Can you work these out from the model? Positions are in its coordinate system, mm. A direction names the side the tool comes from. Coordinates: 2 decimals unless noted, no trailing zeros. Loops run counter-clockwise (first coordinate to the right, second up) from the corner with the lowest first, then second, coordinate; pieces in that order, holes last.
```python
from build123d import *

# Parameters (mm, degrees)
SKETCH1_R               = 8
BOSS_EXTRUDE1_DEPTH     = 1.5
SKETCH2_R               = 6.11
BOSS_EXTRUDE2_DEPTH     = 7
SKETCH4_R               = 8
BOSS_EXTRUDE4_DEPTH     = 7.5
SKETCH6_R               = 4
CUT_EXTRUDE1_DEPTH      = 16
CUT_EXTRUDE2_REACH      = 21.596
CUT_EXTRUDE2_END_RADIUS = 8
SKETCH7_R               = 2.5
CUT_EXTRUDE3_REACH      = 21.596
CUT_EXTRUDE3_END_RADIUS = 8
SKETCH8_R               = 2.5


with BuildPart() as part:
    # Sketch1 → Boss-Extrude1 (new body)
    with BuildSketch(Plane.XY):
        Circle(SKETCH1_R)
    extrude(amount=BOSS_EXTRUDE1_DEPTH)

    # Sketch2 → Boss-Extrude2 (add)
    with BuildSketch(Plane.XY.offset(1.5)):
        Circle(SKETCH2_R)
    extrude(amount=BOSS_EXTRUDE2_DEPTH)

    # Sketch4 → Boss-Extrude4 (add)
    with BuildSketch(Plane.XY.offset(8.5)):
        Circle(SKETCH4_R)
    extrude(amount=BOSS_EXTRUDE4_DEPTH)

    # Sketch6 → Cut-Extrude1 (cut)
    with BuildSketch(Plane.XY.offset(16)):
        Circle(SKETCH6_R)
    extrude(amount=-CUT_EXTRUDE1_DEPTH, mode=Mode.SUBTRACT)

    # Cut-Extrude2: up to this cylinder (the profile starts inside it)
    cut_extrude2_end = Plane(origin=(0, 0, 12.25), z_dir=(0, 0, -1)) * Cylinder(CUT_EXTRUDE2_END_RADIUS, 60.192, mode=Mode.PRIVATE)
    # Sketch7 → Cut-Extrude2 (cut, up to the surface)
    with BuildSketch(Plane.ZY, mode=Mode.PRIVATE) as cut_extrude2_sk1:
        with Locations((12.25, 0)):
            Circle(SKETCH7_R)
    cut_extrude2_tool1 = extrude(cut_extrude2_sk1.sketch, amount=-CUT_EXTRUDE2_REACH, mode=Mode.PRIVATE) & cut_extrude2_end
    add(cut_extrude2_tool1.solids().sort_by_distance((0, 0, 12.25))[0], mode=Mode.SUBTRACT)

    # Cut-Extrude3: up to this cylinder (the profile starts inside it)
    cut_extrude3_end = Plane(origin=(0, 0, 12.25), z_dir=(0, 0, -1)) * Cylinder(CUT_EXTRUDE3_END_RADIUS, 60.192, mode=Mode.PRIVATE)
    # Sketch8 → Cut-Extrude3 (cut, up to the surface)
    with BuildSketch(Plane(origin=(0, 0, 0), x_dir=(0, 0, 1), z_dir=(0, -1, 0)), mode=Mode.PRIVATE) as cut_extrude3_sk1:
        with Locations(Location((12.25, 0, 0), (0, 0, 180))):
            Circle(SKETCH8_R)
    cut_extrude3_tool1 = extrude(cut_extrude3_sk1.sketch, amount=-CUT_EXTRUDE3_REACH, mode=Mode.PRIVATE) & cut_extrude3_end
    add(cut_extrude3_tool1.solids().sort_by_distance((0, 0, 12.25))[0], mode=Mode.SUBTRACT)


solid = part.part
```
(1) If we mould it in two halves opening along Y, with no side actions, what happens to faces 1 (the cylindrical face through (-3.2, -2.4, 8.1)), 2 (the flat face through (-4, -2, 16)), 3 (the cylindrical face through (-1.73, -7.81, 0.74))? For each: released by +Y, released by -Y, zero draft, split by the parting line, or undercut.
Check values:
face 1: undercut
face 2: zero draft
face 3: split by the parting line
(2) I'm going to push flat-ended pins straight in: pin 1 (1 mm diameter, centred on x = 4, z = 10, fed in from -Y); pin 2 (3 mm diameter, centred on y = -5, z = 11.5, fed in from -X); pin 3 (1 mm diameter, centred on y = 4.5, z = 8.5, fed in from -X). Where does each tip first touch, or does it pass through?
Check values:
pin 1: stops at y = -7.19
pin 2: stops at x = -7.19
pin 3: stops at x = -6.93
(3) I want a section at A-A on x = 0. Write out the boundary of the cut face in (y, z).
Check values:
outline: (-8, 0) - (-4, 0) - (-4, 16) - (-8, 16) - (-8, 8.5) - (-6.11, 8.5) - (-6.11, 1.5) - (-8, 1.5) - close; (4, 0) - (8, 0) - (8, 1.5) - (6.11, 1.5) - (6.11, 8.5) - (8, 8.5) - (8, 9.75) - (4, 9.75) - close; (4, 14.75) - (8, 14.75) - (8, 16) - (4, 16) - close
(4) Which directions (+Z, -Z, +X, -X, +Y, -Y) give clear straight access to the entire face, cutting with the end or side of a thin tool? Please do faces 4 (the cylindrical face through (5.53, -2.44, 11.71)), 5 (the cylindrical face through (-2.44, 5.53, 12.79)), 6 (the flat face through (-4, -2, 0)), 7 (the cylindrical face through (-1.73, -7.81, 12.2)), 8 (the flat face through (-2, -6, 1.5)).
Check values:
face 4: +X
face 5: +Y
face 6: -Z, +X, -X, +Y, -Y
face 7: +Z, -Z
face 8: none
(5) If I drill on probe 1 along Z at (x, y) = (6.9, 0); probe 2 along Z at (x, y) = (0, 5.45); probe 3 along Y at (x, z) = (0, 7), over which ranges is the centre line in solid material (lowest first)?
Check values:
probe 1: z = 0 to 1.5, 8.5 to 9.75, 14.75 to 16
probe 2: z = 0 to 9.75, 14.75 to 16
probe 3: y = -6.11 to -4, 4 to 6.11
(6) I want a section at C-C on z = 12.25. Write out the boundary of the cut face in (x, y), then the cut area to 3 significant figures.
Check values:
outline: (-2.5, 3.12) - (-2.5, 7.6) arc R8 ccw (long way) to (7.6, -2.5) - (3.12, -2.5) arc R4 cw (long way) to start; (2.5, 3.12) arc R4 cw to (3.12, 2.5) - (7.6, 2.5) arc R8 ccw to (2.5, 7.6) - close
area: 109 mm2
(7) I want a section at D-D on z = 6.75. Write out the boundary of the cut face in (x, y).
Check values:
outline: circle Ø12.22 at (0, 0); hole circle Ø8 at (0, 0)
